Autodesk Inventor part; units mm, degrees
ref_plane "Work Plane1" through (0, -32.6, 0) normal (0, -1, 0) x (1, 0, 0)
ref_plane "Work Plane2" through (0, 10, 38) normal (1, 0, 0) x (0, 0, -1)
ref_plane "XZ Plane" through (0, 0, 0) normal (0, 1, 0) x (-1, 0, 0)
sketch "Sketch1" plane through (0, 0, 0) normal (1, 0, 0) x (0, 1, 0)
  line L0 (49, 16) -> (63, 16)
  line L1 (63, 16) -> (63, 70)
  line L2 (63, 70) -> (49, 70)
  line L3 (49, 70) -> (49, 16)
  line L4 (63, 16) -> (65, 16)
  line L5 (65, 16) -> (65, 36)
  line L6 (65, 36) -> (63, 36)
  line L7 (63, 36) -> (63, 16)
  line L8 (-65, 0) -> (65, 0) construction
  line L9 (65, 0) -> (49, 0) construction
  line L10 (0, 0) -> (0, 95.8184) construction
  line L11 (-65, 0) -> (-49, 0) construction
  line L12 (0, 0) -> (-21.3713, 0)
  dimension "Lenght" = 130
  dimension "DN" = 32
  dimension "FlgDia" = 140
  dimension "FlgThck" = 16
  dimension "GsktFace" = 72
  dimension "Face" = 2
revolve "Revolution1" add sketch "Sketch1" angle 360 about axis through (0, -65, 0) along (0, 1, 0)
sketch "Sketch5" plane through (0, 63, 0) normal (0, 1, 0) x (1, 0, 0)
  line L0 (0, 0) -> (-35.3553, 35.3553)
  line L1 (0, 0) -> (0, 103.939) construction
  circle A0 centre (-35.3553, 35.3553) radius 9
  point P0 (0, 0)
  dimension "d16" = 50
  dimension "d17" = 45
  dimension "d18" = 18
extrude "Extrusion2" cut sketch "Sketch5" against normal through all
pattern_circular "Circular Pattern1" count 4 over 360 about axis through (0, 64, 0) along (0, 1, 0) of "Extrusion2"
sketch "Sketch14" plane through (0, 49, 0) normal (0, -1, 0) x (-1, 0, 0)
  circle A0 centre (0, 0) radius 16
  circle A1 centre (0, 0) radius 26
  dimension "d54" = 10
pattern_circular "Circular Pattern2" count 2 over 360 about axis through (-10, 0, 0) along (1, 0, 0) of "Revolution1", "Extrusion2", "Circular Pattern1"
extrude "Extrusion5" add sketch "Sketch14" along normal up to surface (98 mm away) contours A0 | A1
sketch "Sketch20" plane through (0, 0, 0) normal (1, 0, 0) x (0, 1, 0)
  line L0 (10, -42.6) -> (10, 42.6)
  arc A0 (10, -42.6) -> (10, 42.6) centre (10, 0) ccw
  line L1 (65, -37.9012) -> (65, 33.7766)
  line L2 (10, 0) -> (18.52, 0)
  line L3 (18.52, 0) -> (18.52, 76)
  line L4 (18.52, 76) -> (10, 76)
  line L5 (10, 76) -> (10, 0)
  line L6 (65, -36) -> (65, 36)
  point P0 (0, 0)
  point P1 (12.4178, -1.9012)
  point P2 (12.4178, -1.9012)
  point P3 (65, -37.9012)
  point P4 (0, 0)
  dimension "d78" = 85.2
  dimension "oI" = 55
  dimension "oH" = 76
  dimension "d81" = 8.52
revolve "Revolution5" add sketch "Sketch20" angle 360 about axis through (0, 10, 76) along (0, 0, -1)
ref_plane "Work Plane1" through (0, -32.6, 0) normal (0, -1, 0) x (1, 0, 0)
sketch "Sketch21" plane through (0, -32.6, 0) normal (0, -1, 0) x (1, 0, 0)
  circle A0 centre (0, 0) radius 26
  circle A1 centre (0, 0) radius 42.5
  point P0 (0, 0)
  dimension "d92" = 85
extrude "Extrusion9" add sketch "Sketch21" against normal blind 16
ref_plane "Work Plane2" through (0, 10, 38) normal (1, 0, 0) x (0, 0, -1)
sketch "Sketch22" plane through (0, 0, 0) normal (0, 1, 0) x (-1, 0, 0)
  line L0 (33, 76) -> (-33, 76)
  line L1 (-33, 76) -> (-33, 163)
  line L2 (-33, 163) -> (33, 163)
  line L3 (33, 163) -> (33, 76)
  line L4 (0, 163) -> (20, 163)
  line L5 (20, 163) -> (20, 183)
  line L6 (20, 183) -> (0, 183)
  line L7 (0, 183) -> (0, 163)
  line L8 (33, 76) -> (-33, 163)
  circle A0 centre (0, 119.5) radius 36
  line L9 (-55.04, 76) -> (0, 76)
  line L10 (-8.52, 76) -> (8.52, 76)
  dimension "oCylWith" = 66
  dimension "oCylHeight" = 87
  dimension "d97" = 20
  dimension "d98" = 20
  dimension "oCylDia" = 72
extrude "Extrusion10" add sketch "Sketch22" along normal mid plane 147 contours A0 L8 L3 | L3 A0 | A0 L1 L8 | A0 L1 picked at (11, 114.7042) picked at (-15.4028, 107.9455)
extrude "Extrusion11" add sketch "Sketch22" along normal mid plane 117 contours L8 A0 L3 | L0 L1 A0 L8 | A0 L8 L3 | A0 L1 L8 | A0 L8 L2 L3 | A0 L1 L8
revolve "Revolution6" add sketch "Sketch22" angle 360 about axis through (0, 0, 183) along (0, 0, -1) contours L2 L7 L6 L5
chamfer "Chamfer1" distance 5 angle 45 4 edges at (-33, 0, 163) (33, 0, 163) (33, 0, 76) (-33, 0, 76)
equation "\"d16\" = 0.5 * KDia"
properties part number "BALL VALVE  PNEUMATIC FLANGED S235 DN32" material "S235"
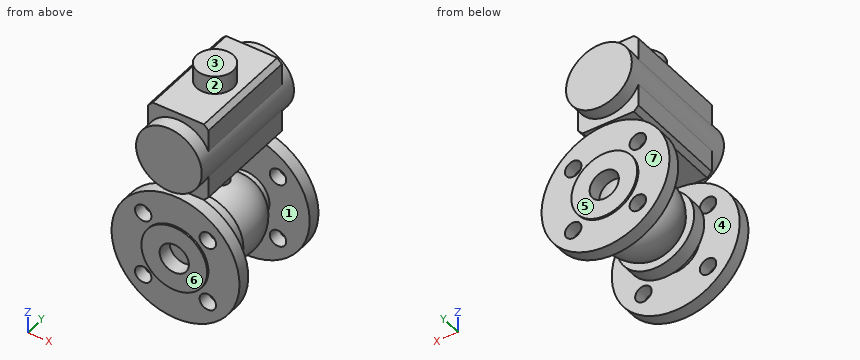
Build history of the part. All positions in model axes, mm. Face numbers are marked on the shaded views. A direction names the side the tool comes from. Give positions to 0.01 mm unless a question says otherwise; leave off trailing zeros. Loops run counter-clockwise (first coordinate to the right, second up) from the corner with the lowest first, then second, coordinate; pieces in that order, holes last. Notation, with made-up numbers: (24.5, 42) - (75.5, 42) arc R27 cw to (75.5, 66) - close; hole circle Ø3 at (-19, -30.5). An arc over 180 degrees is marked (long way). Write item = value, one per line. Start each with the question number.
1) Drop flat-ended pins along their axis: pin 1 Ø5 at (x, y) = (-40.5, 13) entering from +Z; pin 2 Ø2 at (y, z) = (-26, 153) entering from -X; pin 3 Ø12 at (y, z) = (-17.5, 140) entering from +X. Give the stop position or say it passes through.
2) Band-saw the part on A-A on x = -51.5. Give the cut face in (y, z), plus the area to 3 significant figures.
3) Band-saw the part on C-C on y = 35.5. Give the cut face in (x, z), plus the area to 3 significant figures.
4) Band-saw the part on D-D on z = 146. Give the cut face in (x, y).
5) Probe probe 1 along X at (y, z) = (61, 0); probe 2 along Y at (x, z) = (-2, 66); probe 3 along Z at (x, y) = (15, -37). List the from-to ranges inside material, lowest first. Write a range as from..to.
6) Tool access for the marked faces 5, 6 and 7: list every direction of +Z, -Z, +X, -X, +Y, -Y with a clear straight run to the whole face (end or side of a thin tool).
7) Band-saw the part on B-B on z = -54. Give the cut face in (x, y).
8) Pull direction Z, two halves, no side cores. Call the marked faces 1, 2, 3 and 4: +Z half, -Z half, draft (parallel to the pull), parting line (faces both ways), or undercut.
Final values:
q1.pin_1 = 19.03
q1.pin_2 = -33
q1.pin_3 = 33
q2.outline = (-63, -47.41) - (-49, -47.41) - (-49, 47.41) - (-63, 47.41) - close; (49, -47.41) - (63, -47.41) - (63, 47.41) - (49, 47.41) - close
q2.area = 2,650 mm²
q3.outline = circle Ø68.25 at (0, 0); (-33, 81) - (-28, 76) - (28, 76) - (33, 81) - (33, 105.11) arc R36 ccw to (33, 133.89) - (33, 158) - (28, 163) - (-28, 163) - (-33, 158) - (-33, 133.89) arc R36 ccw to (-33, 105.11) - close
q3.area = 9,470 mm²
q4.outline = (-33, -58.5) - (-24.37, -58.5) - (-24.37, -73.5) - (24.37, -73.5) - (24.37, -58.5) - (33, -58.5) - (33, 58.5) - (24.37, 58.5) - (24.37, 73.5) - (-24.37, 73.5) - (-24.37, 58.5) - (-33, 58.5) - close
q5.probe_1 = -70..-16, 16..70
q5.probe_2 = -63..-49, 1.72..18.28, 49..63
q5.probe_3 = -21.24..21.24, 76..163
q6.face_5 = -Z, +X, -X, +Y
q6.face_6 = -Z, +X, -X, -Y
q6.face_7 = +Y
q7.outline = (-44.54, -63) - (44.54, -63) - (44.54, -49) - (-44.54, -49) - close; (-44.54, 49) - (44.54, 49) - (44.54, 63) - (-44.54, 63) - close
q8.face_1 = undercut
q8.face_2 = draft
q8.face_3 = +Z half
q8.face_4 = undercut
